from build123d import *

# Parameters (mm, degrees)
BASPROSKE_W         = 3
BASPROSKE_H         = 16.5
TOOTHCUT_DEPTH      = 24.526580712
TEETHCUTS_COUNT     = 20
TEETHCUTS_ANGLE     = 342
BORSKE_R            = 0.5
BORE_DEPTH          = 50.0000508
SKETCH1_R           = 4.8
BOSS_EXTRUDE1_DEPTH = 3.88
CUT_EXTRUDE1_REACH  = 26.13
SKETCH2_R           = 1.25
SKETCH3_R           = 3
SKETCH3_R_2         = 1.25
CUT_EXTRUDE2_DEPTH  = 1


with BuildPart() as part:
    # BasProSke → Base-Revolve (revolve)
    with BuildSketch(Plane(origin=(0, 0, 0), x_dir=(1, 0, 0), z_dir=(0, 1, 0)), mode=Mode.PRIVATE) as base_revolve_sk:
        with Locations((1.5, 8.25)):
            Rectangle(BASPROSKE_W, BASPROSKE_H)
    revolve(base_revolve_sk.sketch.rotate(Axis((-10, 0, 0), (1, 0, 0)), 180), axis=Axis((-10, 0, 0), (1, 0, 0)))

    # TooCutSke → ToothCut (cut, through all)
    with BuildSketch(Plane(origin=(0, 0, 0), x_dir=(0, 0, -1), z_dir=(1, 0, 0))):
        with BuildLine():
            ThreePointArc((0.74381438, 13.102904875), (0, 13.124), (-0.74381438, 13.102904875))
            ThreePointArc((-0.74381438, 13.102904875), (-1.226473103, 14.852072512), (-2.209965745, 16.376962373))
            ThreePointArc((-2.209965745, 16.376962373), (0, 16.5254), (2.209965745, 16.376962373))
            ThreePointArc((2.209965745, 16.376962373), (1.226473103, 14.852072512), (0.74381438, 13.102904875))
        make_face()
    toothcut = extrude(amount=TOOTHCUT_DEPTH, mode=Mode.SUBTRACT)

    # TeethCuts: ToothCut ×20 about axis
    teethcuts_axis = Axis((-10, 0, 0), (1, 0, 0))
    for i in range(1, TEETHCUTS_COUNT):
        add(toothcut.rotate(teethcuts_axis, i * TEETHCUTS_ANGLE / (TEETHCUTS_COUNT - 1)), mode=Mode.SUBTRACT)

    # BorSke → Bore (cut, symmetric)
    with BuildSketch(Plane(origin=(0, 0, 0), x_dir=(0, 0, -1), z_dir=(1, 0, 0))):
        with Locations(Location((0, 0, 0), (0, 0, 180))):
            Circle(BORSKE_R)
    extrude(amount=BORE_DEPTH, both=True, mode=Mode.SUBTRACT)

    # Sketch1 → Boss-Extrude1 (add)
    with BuildSketch(Plane.ZY):
        with Locations(Location((0, 0, 0), (0, 0, 180))):
            Circle(SKETCH1_R)
        with BuildLine():
            Line((-2.00935313, 1.95), (2.00935313, 1.95))
            ThreePointArc((2.00935313, 1.95), (2.8, 0), (2.00935313, -1.95))
            Line((2.00935313, -1.95), (-2.00935313, -1.95))
            ThreePointArc((-2.00935313, -1.95), (-2.8, 0), (-2.00935313, 1.95))
        make_face(mode=Mode.SUBTRACT)
    extrude(amount=BOSS_EXTRUDE1_DEPTH)

    # Sketch2 → Cut-Extrude1 (cut, up to next)
    with BuildSketch(Plane(origin=(3, 0, 0), x_dir=(0, 0, -1), z_dir=(1, 0, 0)), mode=Mode.PRIVATE) as cut_extrude1_sk1:
        Circle(SKETCH2_R)
    cut_extrude1_tool1 = extrude(cut_extrude1_sk1.sketch, amount=-CUT_EXTRUDE1_REACH, mode=Mode.PRIVATE) & part.part
    add(cut_extrude1_tool1.solids().sort_by_distance((3, 0, 0))[0], mode=Mode.SUBTRACT)

    # Sketch3 → Cut-Extrude2 (cut)
    with BuildSketch(Plane(origin=(3, 0, 0), x_dir=(0, 0, -1), z_dir=(1, 0, 0))):
        Circle(SKETCH3_R)
        Circle(SKETCH3_R_2, mode=Mode.SUBTRACT)
    extrude(amount=-CUT_EXTRUDE2_DEPTH, mode=Mode.SUBTRACT)


solid = part.part
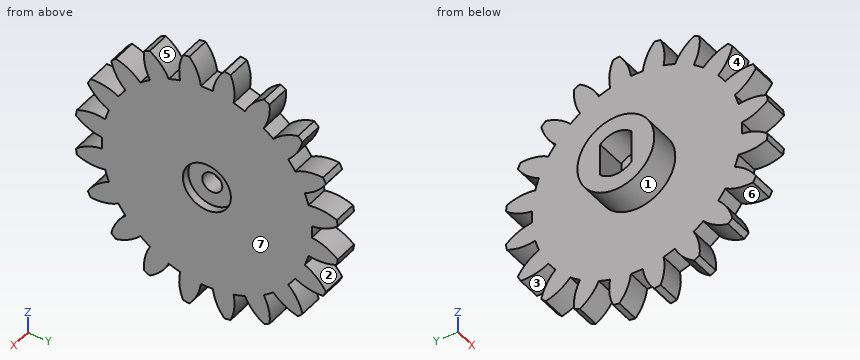
Read the model definition and answer for the solid it produces. Units are mm, in the model's axes. Face numbers are marked on the shaded views. A direction names the side the tool comes from. Give positions to 0.01 mm unless a question says otherwise; leave off trailing zeros. Write each loop counter-clockwise with the first axis right and the second up, starting at its lowest first coordinate (ties: lowest second). Pieces come first, ordered by that corner, then holes. Notation, with made-up numbers: (-25.75, 25) - (-8.75, 25) arc R26 cw to (-8.75, 62) - close; hole circle Ø2 at (-12, 71.5). An arc over 180 degrees is marked (long way). Use CSV: the item, a comma, the result in double quotes. Start each with the question number.
Item 1: The part is cut by section C-C, the plane y = -13.5. Give the vertices of the cut face in (x, z), and give its area (3 significant figures).
Item 2: The part is cut by section A-A, the plane z = 0. Give the vertices of the cut face in (x, y), and give its area (3 significant figures).
Item 3: For the marked faces 1, 2, 3 and 4, determine the directions among +Z, -Z, +X, -X, +Y, -Y from which every point of the face is accessible in a straight line to the end or side of a thin tool.
Item 4: Consider line 1 (Y direction, x = 1.75, z = -11); line 2 (Y direction, x = 2.4, z = 0); line 3 (Y direction, x = 0.7, z = 0). Determine where each line is inside the solid, lowest interval first.
Item 5: The mould has two halves that part along Z. Classify the marked faces 5, 6 and 7: pulls with the +Z half, pulls with the -Z half, needs draft (parallel to the pull), parting line crosses it, or undercut.
Item 6: The part is cut by section D-D, the plane x = -1.5. Give the vertices of the cut face in (y, z), and give its area (3 significant figures).
Item 7: The part is cut by section B-B, the plane y = 0. Give the vertices of the cut face in (x, z), and give its area (3 significant figures).
Item 8: Flat-ended cylindrical pins translate along their axes: P1, Ø1.5, axis at x = 2, y = 7, coming from the +Z side; P2, Ø8, axis at y = 0, z = 0, coming from the -X side; P3, Ø1, axis at x = 2, z = -6.5, coming from the -Y side; P4, Ø3, axis at x = -0.5, z = 12, coming from the +Y side. Find the tip coordinate at first contact, or state that the pin passes through.
Taken from the geometry:
1,outline,"(0, -7.85) - (3, -7.85) - (3, -5.55) - (0, -5.55) - close; (0, -3.45) - (3, -3.45) - (3, -0.8) - (0, -0.8) - close; (0, 0.8) - (3, 0.8) - (3, 3.45) - (0, 3.45) - close; (0, 5.55) - (3, 5.55) - (3, 7.85) - (0, 7.85) - close"
1,area,"29.7 mm2"
2,outline,"(-3.88, -4.8) - (0, -4.8) - (0, -13.12) - (3, -13.12) - (3, -3) - (2, -3) - (2, -1.25) - (0, -1.25) - (0, -1.95) - (-3.88, -1.95) - close; (-3.88, 1.95) - (0, 1.95) - (0, 1.25) - (2, 1.25) - (2, 3) - (3, 3) - (3, 13.12) - (0, 13.12) - (0, 4.8) - (-3.88, 4.8) - close"
2,area,"89.9 mm2"
3,face 1,"-X"
3,face 2,"+X, -X, +Y"
3,face 3,"+X, -X"
3,face 4,"+X, -X, -Y"
4,line 1,"-11.84 to -9.26, -7.16 to 7.16, 9.26 to 11.84"
4,line 2,"-13.12 to -3, 3 to 13.12"
4,line 3,"-13.12 to -1.25, 1.25 to 13.12"
5,face 5,"pulls with the +Z half"
5,face 6,"undercut"
5,face 7,"needs draft"
6,outline,"circle Ø9.6 at (0, 0); hole (-1.95, -2.01) arc R2.8 ccw to (1.95, -2.01) - (1.95, 2.01) arc R2.8 ccw to (-1.95, 2.01) - close"
6,area,"52.5 mm2"
7,outline,"(-3.88, -4.8) - (0, -4.8) - (0, -13.12) - (3, -13.12) - (3, -3) - (2, -3) - (2, -1.25) - (0, -1.25) - (0, -2.8) - (-3.88, -2.8) - close; (-3.88, 2.8) - (0, 2.8) - (0, 1.25) - (2, 1.25) - (2, 3) - (3, 3) - (3, 13.12) - (0, 13.12) - (0, 4.8) - (-3.88, 4.8) - close"
7,area,"83.3 mm2"
8,P1,"z = 14.88"
8,P2,"x = -3.88"
8,P3,"y = -14.79"
8,P4,"y = 11.94"
